Here's how the part is built. I have some questions about the finished solid (model axes, mm). Face numbers are marked on the shaded views. A direction names the side the tool comes from. Round coordinates to 2 decimals unless told otherwise and drop trailing zeros. Write each loop counter-clockwise with the first axis right and the second up, starting at its lowest first coordinate (ties: lowest second). Pieces come first, ordered by that corner, then holes. Notation, with made-up numbers: (14.25, 13) -> (71.25, 13) arc R19 cw to (71.25, 18) -> close; hole circle Ø1 at (43.25, -26). An arc over 180 degrees is marked (long way). Answer as CSV lines item,"result".
from build123d import *

# Parameters (mm, degrees)
SKETCH2_R               = 1.526999994
CUT_EXTRUDE1_DEPTH      = 50.881280215
CUT_EXTRUDE2_DEPTH      = 49.115592108
CUT_EXTRUDE2_DEPTH_BACK = 49.115592108


with BuildPart() as part:
    # Sketch1 → Revolve1 (revolve)
    with BuildSketch(Plane(origin=(0, 0, 0), x_dir=(0, 0, -1), z_dir=(1, 0, 0)), mode=Mode.PRIVATE) as revolve1_sk:
        Polygon((10.999999971, 18.542), (21.999999942, 18.542), (21.999999942, 16.256), (10.999999971, 16.256), (10.999999971, 9.906), (5.999999938, 9.906), (5.999999938, 0), (0, 0), (0, 55.245), (10.999999971, 55.245), align=None)
    revolve(revolve1_sk.sketch.rotate(Axis((0, 55.245, 0), (0, -1, 0)), 180), axis=Axis((0, 55.245, 0), (0, -1, 0)))

    # Sketch2 → Cut-Extrude1 (cut, through all)
    with BuildSketch(Plane.XZ.offset(-16.256)):
        with Locations(Location((0, 17.500000052, 0), (0, 0, 270))):
            Circle(SKETCH2_R)
        with Locations(Location((15.155444611, -8.750000026, 0), (0, 0, 270))):
            Circle(SKETCH2_R)
        with Locations(Location((-15.155444611, -8.750000026, 0), (0, 0, 270))):
            Circle(SKETCH2_R)
    extrude(amount=-CUT_EXTRUDE1_DEPTH, mode=Mode.SUBTRACT)

    # Sketch4 → Cut-Extrude2 (cut, two sides: drawn at the far end of the back side and taken through both)
    with BuildSketch(Plane(origin=(0, 18.542, 0), x_dir=(1, 0, 0), z_dir=(0, 1, 0)).offset(-CUT_EXTRUDE2_DEPTH_BACK)):
        with BuildLine():
            Line((-19.052558833, -10.999999971), (19.052558833, -10.999999971))
            ThreePointArc((19.052558833, -10.999999971), (0, -21.999999942), (-19.052558833, -10.999999971))
        make_face()
    extrude(amount=CUT_EXTRUDE2_DEPTH + CUT_EXTRUDE2_DEPTH_BACK, mode=Mode.SUBTRACT)


solid = part.part
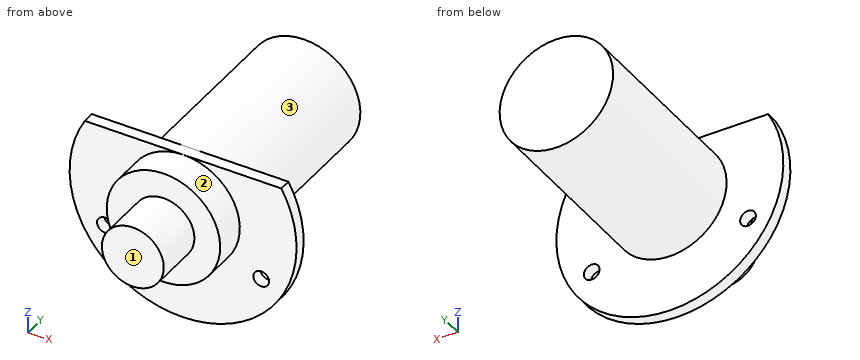
Item 1: Will these pins go through, and if not, where does the flat tip stop? pin 1 (6 mm diameter, centred on x = 4.5, y = 43.5, fed in from -Z); pin 2 (4 mm diameter, centred on y = 17.5, z = -6.5, fed in from -X); pin 3 (4 mm diameter, centred on x = 15.16, z = -8.75, fed in from +Y); pin 4 (6.5 mm diameter, centred on x = -3.5, z = 1, fed in from -Y).
Results found:
pin 1,"stops at z = -10.9"
pin 2,"stops at x = -21.53"
pin 3,"stops at y = 18.54"
pin 4,"stops at y = 0"
Item 2: Suppose I cut it at A-A, the plane z = -8.75. List the corners of the cut face in (x, y) for me (3 decimals).
Results found:
outline,"(-20.185, 16.256) -> (-16.682, 16.256) -> (-16.682, 18.542) -> (-20.185, 18.542) -> close; (-13.628, 16.256) -> (-6.666, 16.256) -> (-6.666, 9.906) -> (6.666, 9.906) -> (6.666, 16.256) -> (13.628, 16.256) -> (13.628, 18.542) -> (6.666, 18.542) -> (6.666, 55.245) -> (-6.666, 55.245) -> (-6.666, 18.542) -> (-13.628, 18.542) -> close; (16.682, 16.256) -> (20.185, 16.256) -> (20.185, 18.542) -> (16.682, 18.542) -> close"
Item 3: For the marked faces 1, 2 and 3, which set-ups out of +Z, -Z, +X, -X, +Y, -Y let a thin tool reach every point of the face, with its end or its side?
Results found:
face 1,"+Z, -Z, +X, -X, -Y"
face 2,"-Y"
face 3,"+Y"
Item 4: Suppose I cut it at B-B, the plane z = 0. List the corners of the cut face in (x, y) for me (3 decimals), then the cut area to 3 significant figures.
Results found:
outline,"(-22, 16.256) -> (-11, 16.256) -> (-11, 9.906) -> (-6, 9.906) -> (-6, 0) -> (6, 0) -> (6, 9.906) -> (11, 9.906) -> (11, 16.256) -> (22, 16.256) -> (22, 18.542) -> (11, 18.542) -> (11, 55.245) -> (-11, 55.245) -> (-11, 18.542) -> (-22, 18.542) -> close"
area,"1,170 mm²"
Item 5: Suppose I cut it at D-D, the plane y = 29. List the corners of the cut face in (x, z) for me.
Results found:
outline,"circle Ø22 at (0, 0)"
Item 6: I need wall thicknesses on L1, parallel to X at y = 17.6, z = -8.75; L2, parallel to X at y = 17, z = -8; L3, parallel to Y at x = 5.5, z = -18. Which ranges of each line are inside material? Lowest first, please.
Results found:
L1,"x = -20.19 to -16.68, -13.63 to 13.63, 16.68 to 20.19"
L2,"x = -20.49 to -16.49, -13.83 to 13.83, 16.49 to 20.49"
L3,"y = 16.26 to 18.54"
Item 7: Suppose I cut it at C-C, the plane x = 7.5. List the corners of the cut face in (y, z) for me (3 decimals), then the cut area to 3 significant figures.
Results found:
outline,"(9.906, -8.047) -> (16.256, -8.047) -> (16.256, -20.682) -> (18.542, -20.682) -> (18.542, -8.047) -> (55.245, -8.047) -> (55.245, 8.047) -> (18.542, 8.047) -> (18.542, 11) -> (16.256, 11) -> (16.256, 8.047) -> (9.906, 8.047) -> close"
area,"765 mm²"
